The listing builds one solid part. Answer for the finished solid, in the listing's coordinates (mm). A direction names the side the tool comes from. Coordinates: 2 decimals unless noted, no trailing zeros. Order: outer loops, then holes, each group sorted by start corner. A loop starts at its lowest first (then second) coordinate and runs counter-clockwise, first axis right, second up. Notation, with made-up numbers: M 66.5,43.5 L 107.5,43.5 A20 ccw 107.5,57.5 Z; hole C 86,-34.75 d4. An arc over 180 degrees is marked long. One line per item, written item: value. Start each with the question number.
Q1. The part is cut by section A-A on z = 20. Give the vertices of the cut face in (x, y).
Q2. Each of these flat-tipped pins is pushed along its axis until it touches: pin 1 Ø9 at (y, z) = (-5.01, 20) entering from -X; pin 2 Ø7.5 at (y, z) = (-2.5, 16) entering from +X; pin 3 Ø6 at (x, z) = (15.5, 28) entering from -Y; pin 4 Ø1.5 at (x, z) = (-3, 32.5) entering from -Y. Where does it stop, or does it pass through?
Q3. The part is cut by section B-B on y = -5. Give the vertices of the cut face in (x, z), then the cut area to 3 significant figures.
Q4. Straight lines are drawn through the part: line 1 along Y through (x, z) = (11.75, 29); line 2 along Y through (x, z) = (-0.5, 34.5); line 3 along X through (y, z) = (8, 29.5). For each, find the intervals that lie inside material, in ascending order. Write a range as [from, to].
Q5. The part is cut by section D-D on z = 26.5. Give the vertices of the cut face in (x, y).
Q6. The part is cut by section C-C on x = 14.25. Give the vertices of the cut face in (y, z).
Q7. Determine the mould class of faces 4 (the flat face through (16, 9.99, 20)), 5 (the cylindrical face through (-6.01, -4.55, 23.47)), 6 (the cylindrical face through (-6.716, 5.689, 20.28)) for opening direction Y: pulls with the +Y half, pulls with the -Y half, needs draft (parallel to the pull), parting line crosses it, or undercut.
Q8. For faces 1 (the flat face through (2, 5, 40)), 2 (the flat face through (-5.001, -1, 20)), 3 (the flat face through (6.999, 9, 20)), determine the directions among +Z, -Z, +X, -X, +Y, -Y from which every point of the face is accessible in a straight line to the end or side of a thin tool.
```python
from build123d import *

# Parameters (mm, degrees)
F1_DEPTH = 40
F2_R     = 1
F3_R     = 5
F4_R     = 3.5
F5_DEPTH = 25
F6_R     = 2
F7_DEPTH = 25
F8_R     = 7


with BuildPart() as f1:
    # F0 (on Top) → F1 (new body)
    with BuildSketch(Plane.XY):
        Polygon((-5.000828, 5.989827), (-7.000828, 5.989827), (-7.000828, -12.010173), (-5.000828, -12.010173), (-5.000828, 3.989827), (6.999172, 3.989827), (8.999172, 3.989827), (8.999172, 9.989827), (21.999172, 9.989827), (21.999172, 11.989827), (8.999172, 11.989827), (6.999172, 11.989827), (6.999172, 9.989827), (6.999172, 5.989827), align=None)
    extrude(amount=F1_DEPTH)

    # F2
    f2_edges = [f1.edges().sort_by_distance(p)[0] for p in [
        (-7.000828, 5.989827, 20),
        (6.999172, 11.989827, 20),
        (-5.000828, 3.989827, 20),
        (8.999172, 9.989827, 20),
        (8.999172, 3.989827, 20),
        (6.999172, 5.989827, 20),
    ]]
    fillet(f2_edges, radius=F2_R)

    # F3
    f3_edges = [f1.edges().sort_by_distance(p)[0] for p in [
        (-6.000828, -12.010173, 0),
        (-6.000828, -12.010173, 40),
    ]]
    fillet(f3_edges, radius=F3_R)

    # F4 (on face) → F5 (cut)
    with BuildSketch(Plane(origin=(-7.000828, 0, 0), x_dir=(0, -1, 0), z_dir=(-1, 0, 0))):
        with Locations((5.010173, 20)):
            Circle(F4_R)
    extrude(amount=-F5_DEPTH, mode=Mode.SUBTRACT)

    # F6 (on face) → F7 (cut)
    with BuildSketch(Plane(origin=(0, 11.989827, 0), x_dir=(-1, 0, 0), z_dir=(0, 1, 0))):
        with Locations((-13.999172, 8)):
            Circle(F6_R)
        with Locations((-13.999172, 32)):
            Circle(F6_R)
    extrude(amount=-F7_DEPTH, mode=Mode.SUBTRACT)

    # F8
    f8_edges = [f1.edges().sort_by_distance(p)[0] for p in [
        (21.999172, 10.989827, 0),
        (21.999172, 10.989827, 40),
    ]]
    fillet(f8_edges, radius=F8_R)


solid = f1.part
```
Output:
1. outline: M -7,-12.01 L -5,-12.01 L -5,-8.51 L -7,-8.51 Z; M -7,-1.51 L -5,-1.51 L -5,2.99 A1 cw -4,3.99 L 8,3.99 A1 ccw 9,4.99 L 9,8.99 A1 cw 10,9.99 L 22,9.99 L 22,11.99 L 8,11.99 A1 ccw 7,10.99 L 7,6.99 A1 cw 6,5.99 L -6,5.99 A1 ccw -7,4.99 Z
2. pin 1: stops at x = -7
2. pin 2: stops at x = -5
2. pin 3: stops at y = 9.99
2. pin 4: stops at y = 3.99
3. outline: M -7,0 L -5,0 L -5,16.5 L -7,16.5 Z; M -7,23.5 L -5,23.5 L -5,40 L -7,40 Z
3. area: 66.0 mm^2
4. line 1: y = [9.99, 11.99]
4. line 2: y = [3.99, 5.99]
4. line 3: x = [7, 9]
5. outline: M -7,-12.01 L -5,-12.01 L -5,2.99 A1 cw -4,3.99 L 8,3.99 A1 ccw 9,4.99 L 9,8.99 A1 cw 10,9.99 L 22,9.99 L 22,11.99 L 8,11.99 A1 ccw 7,10.99 L 7,6.99 A1 cw 6,5.99 L -6,5.99 A1 ccw -7,4.99 Z
6. outline: M 9.99,0 L 11.99,0 L 11.99,6.02 L 9.99,6.02 Z; M 9.99,9.98 L 11.99,9.98 L 11.99,30.02 L 9.99,30.02 Z; M 9.99,33.98 L 11.99,33.98 L 11.99,40 L 9.99,40 Z
7. face 4: pulls with the -Y half
7. face 5: undercut
7. face 6: pulls with the +Y half
8. face 1: +Z, +X, -X, +Y, -Y
8. face 2: +Z, -Z, +X, -Y
8. face 3: +Z, -Z, -X, +Y
